Answer from the drawing. Dimensions are ordinates in mm from the lowest x, y and z of the part. Give positions to 0.01 mm unless a question says otherwise; leave off trailing zeros. Loops run counter-clockwise (first coordinate to the right, second up) from the corner with the lowest first, then second, coordinate; pieces in that order, holes last. Notation, with made-up numbers: M 2.5,-29.5 L 37.5,-29.5 A31 cw 37.5,5.5 Z; hole C 31.25,-7 d8. An arc over 180 degrees is marked long. Use a Markdown table: item, result.
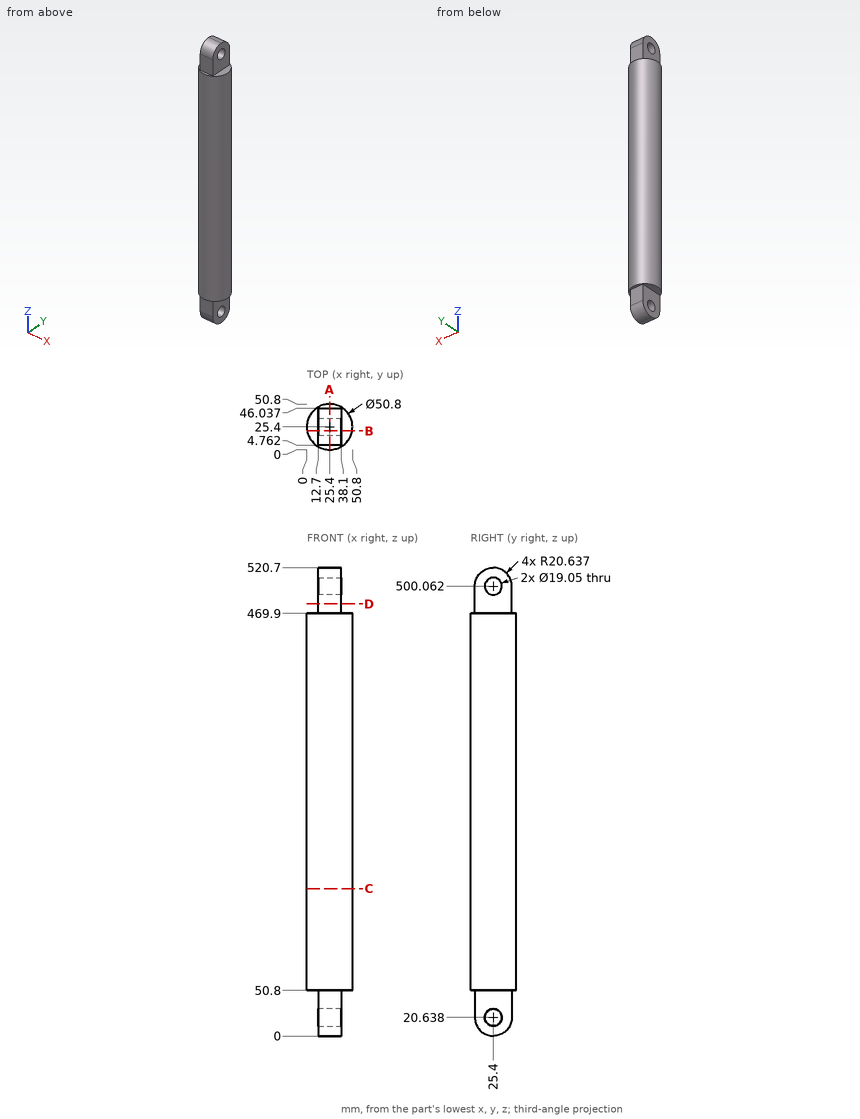
(1) A cutting plane is placed at B-B (y = 21). Write down the section's boundary in (x, z) (1 decimal).
Entries:
| item | result |
|---|---|
| outline | M 0.4,50.8 L 12.7,50.8 L 12.7,29.1 L 38.1,29.1 L 38.1,50.8 L 50.4,50.8 L 50.4,469.9 L 38.1,469.9 L 38.1,491.6 L 12.7,491.6 L 12.7,469.9 L 0.4,469.9 Z; M 12.7,0.5 L 38.1,0.5 L 38.1,12.2 L 12.7,12.2 Z; M 12.7,508.5 L 38.1,508.5 L 38.1,520.2 L 12.7,520.2 Z |
(2) A cutting plane is placed at C-C (z = 164). Write down the section's boundary in (x, y).
Entries:
| item | result |
|---|---|
| outline | C 25.4,25.4 d50.8 |
(3) Given P1, Ø5, axis at x = 14.5, z = 212, coming from the -Y side; P2, Ø10, axis at x = 41.5, z = 148.5, coming from the +Y side (1 decimal); P3, Ø5, axis at x = 14, z = 239, coming from the -Y side, each flat-ended and moving along its own axis, determine where each tip first touches the part or whether it passes through.
Entries:
| item | result |
|---|---|
| P1 | stops at y = 1.43 |
| P2 | stops at y = 48.2 |
| P3 | stops at y = 1.61 |
(4) A cutting plane is placed at D-D (z = 480.5). Write down the section's boundary in (x, y).
Entries:
| item | result |
|---|---|
| outline | M 12.7,4.76 L 38.1,4.76 L 38.1,46.04 L 12.7,46.04 Z |
(5) Consider probe 1 along Z at (x, y) = (33.5, 29.5) (1 decimal); probe 2 along Z at (x, y) = (32.5, 32) (1 decimal); probe 3 along X at (y, z) = (12, 471). Determine where each line is inside the solid, lowest interval first. Write a range as [from, to].
Entries:
| item | result |
|---|---|
| probe 1 | z = [0.4, 12], [29.2, 491.5], [508.7, 520.3] |
| probe 2 | z = [1.1, 13.8], [27.5, 493.2], [506.9, 519.6] |
| probe 3 | x = [12.7, 38.1] |
(6) A cutting plane is placed at A-A (x = 25.4). Count the separate pieces of the cut face and the enclosed holes in it, and give its area (3 significant figures).
Entries:
| item | result |
|---|---|
| separate pieces | 1 |
| enclosed holes | 2 |
| area | 24,500 mm² |
